```python
from build123d import *

# Parameters (mm, degrees)
BASE_BODY_DEPTH      = 7.9375
BASE_BODY_DEPTH_BACK = 7.9375


with BuildPart() as part:
    # Sketch36 → base body (new, two sides: drawn at the far end of the back side and taken through both)
    with BuildSketch(Plane(origin=(20.921737804, 196.649439362, -18.857828861), x_dir=(-0.9944387813726006, 0.10483531003395151, -0.010053251825273378), z_dir=(-0.10531623854931917, -0.9898976586232768, 0.09492689476632808)).offset(-BASE_BODY_DEPTH_BACK)):
        with BuildLine():
            Line((502.126358952, -759.009489392), (509.776945736, -773.997260344))
            Line((509.776945736, -773.997260344), (553.695188941, -751.57896131))
            Line((553.695188941, -751.57896131), (566.064134599, -750.762637468))
            ThreePointArc((566.064134599, -750.762637468), (571.160491163, -749.431075239), (575.401507546, -746.307025266))
            Line((575.401507546, -746.307025266), (579.083820389, -735.902974553))
            Line((579.083820389, -735.902974553), (574.066112376, -726.073106528))
            ThreePointArc((574.066112376, -726.073106528), (569.451308261, -723.533521683), (564.224157475, -722.883288763))
            Line((564.224157475, -722.883288763), (551.855211817, -723.699612605))
            Line((551.855211817, -723.699612605), (507.741248901, -708.086327289))
            Line((507.741248901, -708.086327289), (502.126762386, -723.949564583))
            Line((502.126762386, -723.949564583), (502.126358952, -759.009489392))
        make_face()
    extrude(amount=BASE_BODY_DEPTH + BASE_BODY_DEPTH_BACK)


solid = part.part
```
Check sheet for the modelled part. Datum: model origin and axes. Units: mm. Round coordinates to 2 decimals unless told otherwise and drop trailing zeros. Loops run counter-clockwise (first coordinate to the right, second up) from the corner with the lowest first, then second, coordinate; pieces in that order, holes last. Notation, with made-up numbers: M 44.5,29.5 L 100.5,29.5 A15 ccw 100.5,52.5 Z; hole C 84,87 d10. An arc over 180 degrees is marked long. Answer as a JSON object with one key per item and string values.
1. Section check A-A (x = -536). Record the boundary of the cut face in (y, z).
Reply:
{"outline": "M 316.45,696.19 L 332.33,694.55 L 335.01,722.43 L 319.12,724.06 Z"}
2. Section check B-B (z = 734). Record the boundary of the cut face in (x, y).
Reply:
{"outline": "M -512.25,317.55 L -480.07,314.13 L -479.17,330.07 L -507.69,333.1 Z"}
3. Mould release check, pull along X, two halves, no side actions. Record for faces 1 (the flat face through (-534.089, 324.314, 695.503)), 2 (the flat face through (-508.474, 315.208, 713.751)), 3 (the flat face through (-506.8, 330.92, 712.24)): pulls with the +X half, pulls with the -X half, needs draft (parallel to the pull), parting line crosses it, or undercut.
Reply:
{"face 1": "undercut", "face 2": "pulls with the -X half", "face 3": "pulls with the +X half"}
4. Gauge pin test, flat ends, axial feed: P1, Ø2, axis at y = 322.5, z = 714, coming from the -X side; P2, Ø10, axis at y = 314, z = 714.5, coming from the +X side; P3, Ø8, axis at x = -530, z = 712, coming from the +Y side; P4, Ø5, axis at x = -529.5, z = 729.5, coming from the -Y side. Record the tip position at first contact, or that the pin passes through.
Reply:
{"P1": "stops at x = -553.91", "P2": "stops at x = -478.53", "P3": "stops at y = 333.94", "P4": "passes through"}
5. Scan lines: line 1 (X direction, y = 326.5, z = 728); line 2 (Z direction, x = -524.5, y = 330.5); line 3 (Y direction, x = -497, z = 736.5). Record each from-to range of solid material in increasing order.
Reply:
{"line 1": "x = -521.33 to -477.87", "line 2": "z = 694.4 to 725.77", "line 3": "y = 316.17 to 332.21"}
